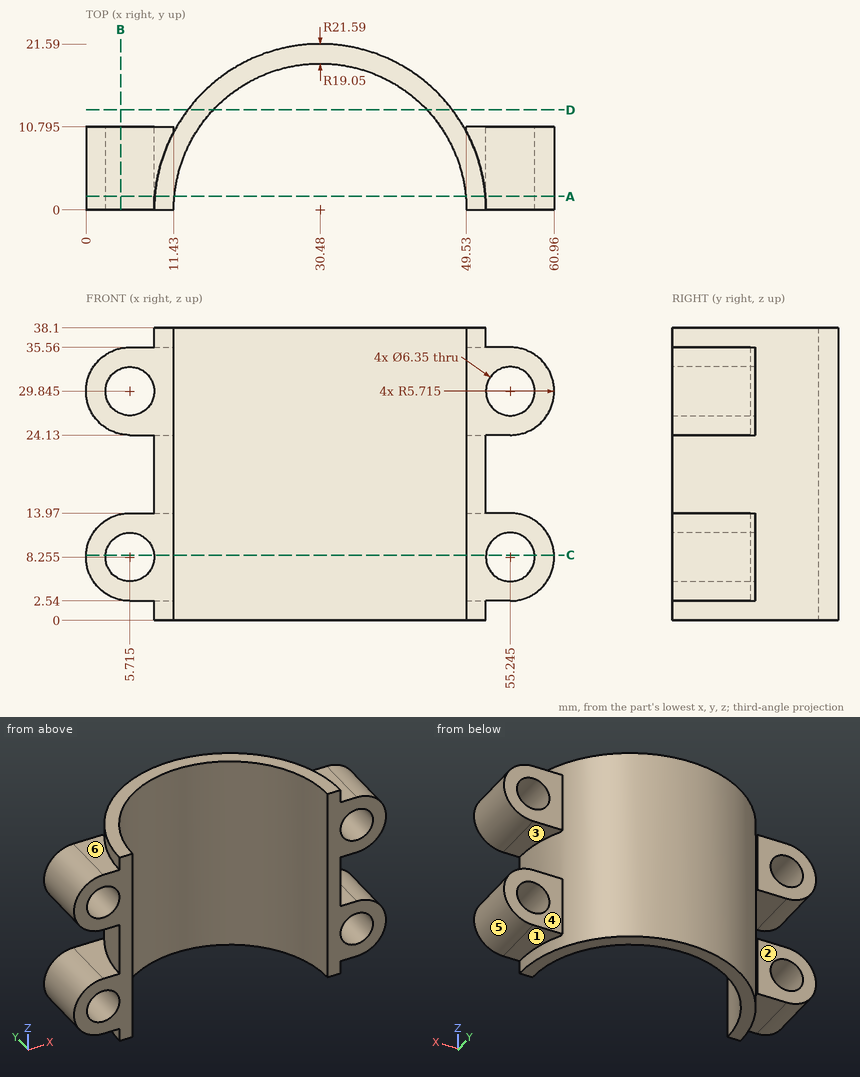
Print and shaded views of the part. All mm, measured from the part's lowest x, y and z. A direction names the side the tool comes from. Coordinates: 2 decimals unless noted, no trailing zeros. Write each loop counter-clockwise with the first axis right and the second up, starting at its lowest first coordinate (ties: lowest second). Pieces come first, ordered by that corner, then holes. Notation, with made-up numbers: M -39,14 L 20,14 A15 ccw 20,32 Z; hole C 23,24 d4. An arc over 180 degrees is marked long. Return JSON: item names as keys, results as strings.
1. Saw through at D-D, the plane y = 13. Write the cut outline in (x, z), then the cut area to 3 significant figures.
Determined:
{"outline": "M 13.24,0 L 16.56,0 L 16.56,38.1 L 13.24,38.1 Z; M 44.4,0 L 47.72,0 L 47.72,38.1 L 44.4,38.1 Z", "area": "252 mm²"}
2. Flat gauge pins, fed straight in: pin 1 Ø7.5 at (x, z) = (55.245, 29.845) entering from +Y (3 decimals); pin 2 Ø0.5 at (y, z) = (10.5, 5.5) entering from +X; pin 3 Ø5 at (y, z) = (18.5, 11) entering from -X. Where does each tip first touch, or does it go through?
Determined:
{"pin 1": "y = 10.795", "pin 2": "x = 60.38", "pin 3": "x = 15.98"}
3. Pull direction Z, two halves, no side cores. Call the marked faces 4, 5 and 6: pulls with the +Z half, pulls with the -Z half, needs draft (parallel to the pull), parting line crosses it, or undercut.
Determined:
{"face 4": "needs draft", "face 5": "undercut", "face 6": "pulls with the +Z half"}
4. 3-axis set-ups, long thin cutter, end or side, ignore diameter. For the marked faces 1, 2 and 3: which of +Z, -Z, +X, -X, +Y, -Y reach the whole face in a straight line?
Determined:
{"face 1": "-Z, +X, +Y", "face 2": "+Z, -Z, -X, +Y", "face 3": "+X, +Y"}
5. Saw through at C-C, the plane z = 8.5. Write the cut outline in (x, y) (3 decimals).
Determined:
{"outline": "M 0.005,0 L 2.549,0 L 2.549,10.795 L 0.005,10.795 Z; M 8.881,0 L 11.43,0 A19.05 cw 49.53,0 L 52.079,0 L 52.079,10.795 L 49.53,10.795 L 49.53,10.16 A21.59 ccw 11.43,10.16 L 11.43,10.795 L 8.881,10.795 Z; M 58.411,0 L 60.955,0 L 60.955,10.795 L 58.411,10.795 Z"}
6. Saw through at B-B, the plane x = 4.5. Write the cut outline in (y, z) (3 decimals), then the cut area to 3 significant figures.
Determined:
{"outline": "M 0,2.671 L 10.795,2.671 L 10.795,5.322 L 0,5.322 Z; M 0,11.188 L 10.795,11.188 L 10.795,13.839 L 0,13.839 Z; M 0,24.261 L 10.795,24.261 L 10.795,26.912 L 0,26.912 Z; M 0,32.778 L 10.795,32.778 L 10.795,35.429 L 0,35.429 Z", "area": "114 mm²"}
7. Saw through at A-A, the plane y = 1.75. Write the cut outline in (x, z) (3 decimals).
Determined:
{"outline": "M 5.715,2.54 L 8.961,2.54 L 8.961,0 L 11.511,0 L 11.511,38.1 L 8.961,38.1 L 8.961,35.56 L 5.715,35.56 A5.715 ccw 5.715,24.13 L 8.961,24.13 L 8.961,13.97 L 5.715,13.97 A5.715 ccw Z; M 49.449,0 L 51.999,0 L 51.999,2.54 L 55.245,2.54 A5.715 ccw 55.245,13.97 L 51.999,13.97 L 51.999,24.13 L 55.245,24.13 A5.715 ccw 55.245,35.56 L 51.999,35.56 L 51.999,38.1 L 49.449,38.1 Z; hole C 5.715,8.255 d6.35; hole C 5.715,29.845 d6.35; hole C 55.245,8.255 d6.35; hole C 55.245,29.845 d6.35"}
8. Probe L1, parallel to Y at x = 51, z = 35.5 (3 decimals); L2, parallel to X at y = 8.5, z = 18; L3, parallel to X at y = 8, z = 11.5. List the from-to ranges inside material, lowest first.
Determined:
{"L1": "0 to 10.795", "L2": "10.63 to 13.43, 47.53 to 50.33", "L3": "1.01 to 13.19, 47.77 to 59.95"}
